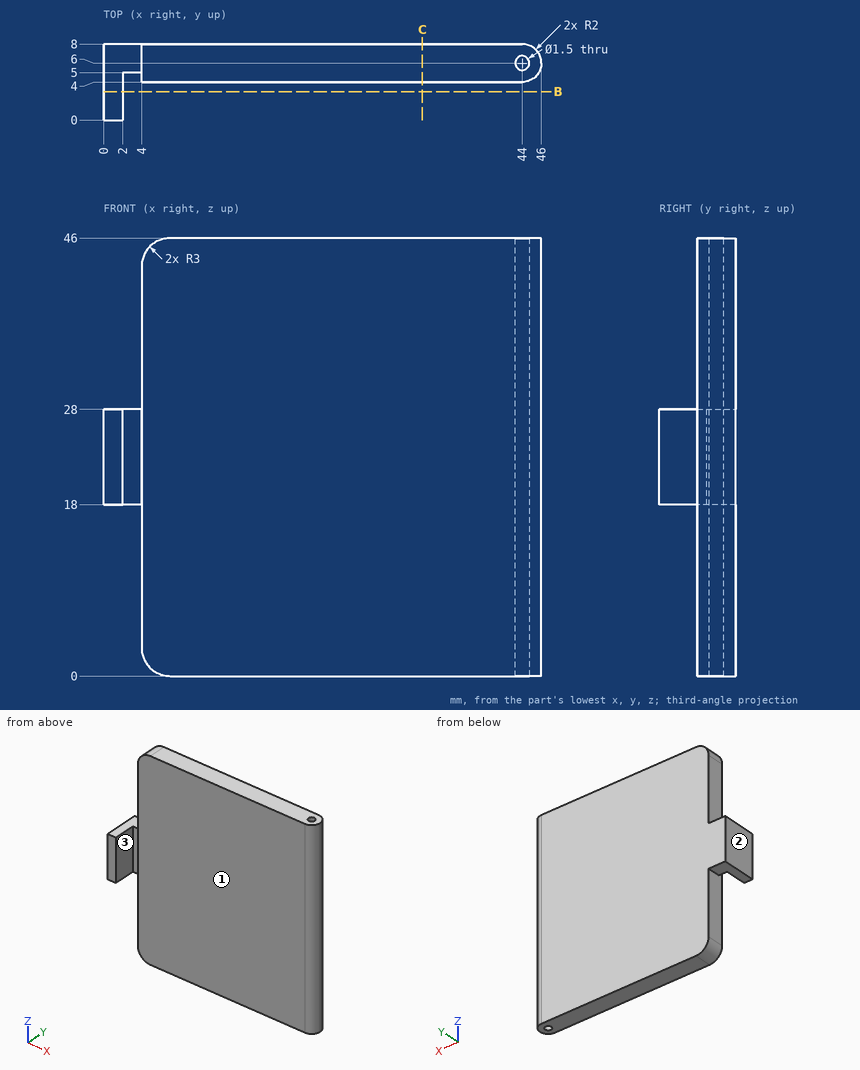
Input: dimensioned drawing with shaded views. Units: mm. Origin: part minimum x, y, z. A direction names the side the tool comes from. Coordinates: 2 decimals unless noted, no trailing zeros. Write each loop counter-clockwise with the first axis right and the second up, starting at its lowest first coordinate (ties: lowest second). Pieces come first, ordered by that corner, then holes. Notation, with made-up numbers: (22, -12.5) -> (43, -12.5) arc R21 ccw to (43, 25.5) -> close; hole circle Ø8 at (84.25, -7). An arc over 180 degrees is marked (long way). Return JSON: item names as keys, results as strings. Group by question number.
1) Section query C-C, the plane x = 33.5. Return loops of the section in (y, z).
2) Set-up query: the marked faces 1, 2 and 3. Return all of +Z, -Z, +X, -X, +Y, -Y with unobstructed straight access to the full face (end or side cutting, diameter ignored); none if empty.
3) Ray query, line 1 along Y through (x, z) = (44, 11.5); line 2 along Y through (x, z) = (10.5, 15); line 3 along Z through (x, y) = (3, 7.75). Return the intervals inside material, ascending.
4) Section query B-B, the plane y = 3. Return loops of the section in (x, z), plus the area to 3 significant figures.
5) Contact query for flat-ended pins moving along their axis: P1, Ø3, axis at x = 39, z = 28.5, coming from the -Y side; P2, Ø1.5, axis at y = 2.5, z = 22.5, coming from the +X side; P3, Ø1.2, axis at x = 1, y = 2, coming from the -Z side. Output: stop coordinate, or through.
From the geometry:
{
 "1": {"outline": "(4, 0) -> (8, 0) -> (8, 46) -> (4, 46) -> close"},
 "2": {"face 1": "+Z, -Z, +X, -Y", "face 2": "+Z, -Z, -X, +Y, -Y", "face 3": "+Z, -Z, -Y"},
 "3": {"line 1": "4 to 5.25, 6.75 to 8", "line 2": "4 to 8", "line 3": "18 to 28"},
 "4": {"outline": "(0, 18) -> (2, 18) -> (2, 28) -> (0, 28) -> close", "area": "20.0 mm²"},
 "5": {"P1": "y = 4", "P2": "x = 2", "P3": "z = 18"}
}
